from build123d import *

# Parameters (mm, degrees)
SKETCH1_R           = 24.13
SKETCH1_R_2         = 21.43125
BOSS_EXTRUDE1_DEPTH = 25.4
SKETCH2_W           = 6.223
SKETCH2_H           = 31.914566101
CUT_EXTRUDE1_DEPTH  = 25.4
CIRPATTERN1_COUNT   = 4
SKETCH3_R           = 24.13
SKETCH3_R_2         = 21.43125
BOSS_EXTRUDE3_DEPTH = 3.175
SKETCH4_R           = 49.609375
SKETCH4_R_2         = 24.13
BOSS_EXTRUDE4_DEPTH = 3.175
BOSS_EXTRUDE5_DEPTH = 25.4
SKETCH11_R          = 21.43125
SKETCH11_R_2        = 20.955
BOSS_EXTRUDE6_DEPTH = 28.575
SKETCH14_R          = 49.609375
SKETCH14_R_2        = 20.955
BOSS_EXTRUDE7_DEPTH = 3.175
SKETCH15_W          = 94.553098484
SKETCH15_H          = 6.29591516
CUT_EXTRUDE8_DEPTH  = 25.4
SKETCH16_W          = 6.29591516
SKETCH16_H          = 94.553098484
CUT_EXTRUDE9_DEPTH  = 25.4


with BuildPart() as part:
    # Sketch1 → Boss-Extrude1 (new body)
    with BuildSketch(Plane(origin=(0, 0, 0), x_dir=(1, 0, 0), z_dir=(0, 1, 0))):
        Circle(SKETCH1_R)
        Circle(SKETCH1_R_2, mode=Mode.SUBTRACT)
    extrude(amount=BOSS_EXTRUDE1_DEPTH)

    # Sketch2 → Cut-Extrude1 (cut)
    with BuildSketch(Plane.XY):
        with Locations((0, 15.957283051)):
            Rectangle(SKETCH2_W, SKETCH2_H)
    cut_extrude1 = extrude(amount=-CUT_EXTRUDE1_DEPTH, mode=Mode.SUBTRACT)

    # CirPattern1: Cut-Extrude1 ×4 about axis
    cirpattern1_axis = Axis((0, 0, 0), (0, 1, 0))
    for i in range(1, CIRPATTERN1_COUNT):
        add(cut_extrude1.rotate(cirpattern1_axis, i * 360 / CIRPATTERN1_COUNT), mode=Mode.SUBTRACT)

    # Sketch3 → Boss-Extrude3 (add)
    with BuildSketch(Plane.XZ):
        Circle(SKETCH3_R)
        Circle(SKETCH3_R_2, mode=Mode.SUBTRACT)
    extrude(amount=BOSS_EXTRUDE3_DEPTH)

    # Sketch4 → Boss-Extrude4 (add)
    with BuildSketch(Plane(origin=(0, -3.175, 0), x_dir=(-1, 0, 0), z_dir=(0, -1, 0))):
        Circle(SKETCH4_R)
        Circle(SKETCH4_R_2, mode=Mode.SUBTRACT)
    extrude(amount=-BOSS_EXTRUDE4_DEPTH)

    # Sketch6 → Boss-Extrude5 (add)
    with BuildSketch(Plane(origin=(0, 0, 0), x_dir=(1, 0, 0), z_dir=(0, 1, 0))):
        Polygon((3.1115, 21.204175162), (3.1115, 23.929621576), (3.1115, 47.249506822), (6.35, 47.249506822), (6.35, 22.127823022), align=None)
        Polygon((-3.1115, 21.204175162), (-3.1115, 23.929621576), (-3.1115, 47.249506822), (-6.35, 47.249506822), (-6.35, 22.127823022), align=None)
        Polygon((21.267675162, 3.12091516), (23.993121576, 3.12091516), (47.313006822, 3.12091516), (47.313006822, 6.35941516), (22.191323022, 6.35941516), align=None)
        Polygon((47.313006822, -3.10208484), (23.993121576, -3.10208484), (21.267675162, -3.10208484), (22.191323022, -6.34058484), (47.313006822, -6.34058484), align=None)
        Polygon((3.18441516, -21.258260002), (3.18441516, -23.983706416), (3.18441516, -47.303591662), (6.42291516, -47.303591662), (6.42291516, -22.181907862), align=None)
        Polygon((-3.03858484, -47.303591662), (-3.03858484, -23.983706416), (-3.03858484, -21.258260002), (-6.27708484, -22.181907862), (-6.27708484, -47.303591662), align=None)
        Polygon((-21.194760002, -3.175), (-23.920206416, -3.175), (-47.240091662, -3.175), (-47.240091662, -6.4135), (-22.118407862, -6.4135), align=None)
        Polygon((-47.240091662, 3.048), (-23.920206416, 3.048), (-21.194760002, 3.048), (-22.118407862, 6.2865), (-47.240091662, 6.2865), align=None)
    extrude(amount=BOSS_EXTRUDE5_DEPTH)

    # Sketch11 → Boss-Extrude6 (add)
    with BuildSketch(Plane.XZ.offset(3.175)):
        Circle(SKETCH11_R)
        Circle(SKETCH11_R_2, mode=Mode.SUBTRACT)
    extrude(amount=-BOSS_EXTRUDE6_DEPTH)

    # Sketch14 → Boss-Extrude7 (add)
    with BuildSketch(Plane.XZ.offset(3.175)):
        Circle(SKETCH14_R)
        Circle(SKETCH14_R_2, mode=Mode.SUBTRACT)
    extrude(amount=BOSS_EXTRUDE7_DEPTH)

    # Sketch15 → Cut-Extrude8 (cut)
    with BuildSketch(Plane(origin=(0, 25.4, 0), x_dir=(1, 0, 0), z_dir=(0, 1, 0))):
        with Locations((0.03645758, -0.02704242)):
            Rectangle(SKETCH15_W, SKETCH15_H)
    extrude(amount=-CUT_EXTRUDE8_DEPTH, mode=Mode.SUBTRACT)

    # Sketch16 → Cut-Extrude9 (cut)
    with BuildSketch(Plane(origin=(0, 25.4, 0), x_dir=(1, 0, 0), z_dir=(0, 1, 0))):
        with Locations((0.03645758, -0.02704242)):
            Rectangle(SKETCH16_W, SKETCH16_H)
    extrude(amount=-CUT_EXTRUDE9_DEPTH, mode=Mode.SUBTRACT)


solid = part.part
CAD build for the part. Positions are in the model's coordinates, mm. A direction names the side the tool comes from. Give positions to 0.01 mm unless a question says otherwise; leave off trailing zeros. Order: outer loops, then holes, each group sorted by start corner. A loop starts at its lowest first (then second) coordinate and runs counter-clockwise, first axis right, second up. Notation, with made-up numbers: (84, 46) - (121, 46) arc R6 cw to (121, 53) - close; hole circle Ø3 at (-33.5, 89). An arc over 180 degrees is marked (long way). Answer in a Markdown table with one row per item.
1. Tool access for faces 1 (the flat face through (-47.24, 13, -5)), 2 (the flat face through (34, 13, 3.175)), 3 (the flat face through (6.423, 13, 35)), 4 (the cylindrical face through (-17.209, 12.878, -16.914)), 5 (the flat face through (-35, 13, 6.414)): list every direction of +Z, -Z, +X, -X, +Y, -Y with a clear straight run to the whole face (end or side of a thin tool).
Data:
| item | result |
|---|---|
| face 1 | +Z, -Z, -X, +Y |
| face 2 | +X, -X, +Y |
| face 3 | +Z, +X, +Y |
| face 4 | -Z, -X, +Y |
| face 5 | +Z, -X, +Y |
2. Pull direction X, two halves, no side cores. Call faces 6 (the flat face through (-5, 13, -47.25)), 7 (the cylindrical face through (17.216, 12.878, 16.908)), 8 (the flat face through (3.184, 13, -34)): pulls with the +X half, pulls with the -X half, needs draft (parallel to the pull), parting line crosses it, or undercut.
Data:
| item | result |
|---|---|
| face 6 | needs draft |
| face 7 | pulls with the +X half |
| face 8 | undercut |
3. Flat gauge pins, fed straight in: pin 1 (1 mm diameter, centred on x = -4.5, y = 17, fed in from -Z); pin 2 (3 mm diameter, centred on x = 19.5, y = 2, fed in from +Z); pin 3 (1.6 mm diameter, centred on y = 12.5, z = -4, fed in from +X). Where does each tip first touch, or does it go through?
Data:
| item | result |
|---|---|
| pin 1 | stops at z = -47.25 |
| pin 2 | stops at z = 16.07 |
| pin 3 | stops at x = 47.31 |
4. Probe probe 1 along Z at (x, y) = (42, 15) (3 decimals); probe 2 along Z at (x, y) = (0, -4.3) (3 decimals); probe 3 along X at (y, z) = (19.5, -41). List the from-to ranges inside material, lowest first. Write a range as [from, to].
Data:
| item | result |
|---|---|
| probe 1 | z = [-6.359, -3.121], [3.175, 6.341] |
| probe 2 | z = [-49.609, -20.955], [20.955, 49.609] |
| probe 3 | x = [-6.35, -3.11], [3.18, 6.35] |
5. Saw through at C-C, the plane x = 0. Give the cut face in (y, z) (3 decimals), plus the area to 3 significant figures.
Data:
| item | result |
|---|---|
| outline | (-6.35, -49.609) - (0, -49.609) - (0, -20.955) - (-6.35, -20.955) - close; (-6.35, 20.955) - (0, 20.955) - (0, 49.609) - (-6.35, 49.609) - close |
| area | 364 mm² |
6. Saw through at B-B, the plane y = 14. Count the separate pieces of the cut face and the enclosed holes in it, plus the area to 3 significant figures.
Data:
| item | result |
|---|---|
| separate pieces | 4 |
| enclosed holes | 0 |
| area | 975 mm² |
7. Saw through at A-A, the plane z = 0. Give the cut face in (x, y) (3 decimals), plus the area to 3 significant figures.
Data:
| item | result |
|---|---|
| outline | (-49.609, -6.35) - (-20.955, -6.35) - (-20.955, 0) - (-49.609, 0) - close; (20.955, -6.35) - (49.609, -6.35) - (49.609, 0) - (20.955, 0) - close |
| area | 364 mm² |
